Work out the finished part from the listing and answer in its coordinate system (mm). A direction names the side the tool comes from. Round coordinates to 2 decimals unless told otherwise and drop trailing zeros. Write each loop counter-clockwise with the first axis right and the second up, starting at its lowest first coordinate (ties: lowest second). Pieces come first, ordered by that corner, then holes. Notation, with made-up numbers: (-37.5, 13) -> (10.5, 13) arc R19 ccw to (10.5, 36) -> close; hole circle Ø6 at (54, -39.75). An arc over 180 degrees is marked (long way). One line per question, with ' | ' between items. Start each with the question number.
```python
from build123d import *

# Parameters (mm, degrees)
ESQUISSE1_W             = 41.6
ESQUISSE1_H             = 40
BOSS_EXTRU_1_DEPTH      = 4
BOSS_EXTRU_2_DEPTH      = 20
ESQUISSE3_R             = 19
ENL_V_MAT_EXTRU_1_DEPTH = 15
ENL_V_MAT_EXTRU_2_REACH = 62.626
ESQUISSE5_R             = 7
BOSS_EXTRU_3_DEPTH      = 6
D_GAGEMENT_M31_D        = 3.6
CONG_1_R                = 10
D_GAGEMENT_M32_D        = 3.6
ENL_V_MAT_EXTRU_3_DEPTH = 2.4
CONG_2_R                = 2


with BuildPart() as part:
    # Esquisse1 → Boss.-Extru.1 (new body)
    with BuildSketch(Plane(origin=(0, 0, 0), x_dir=(1, 0, 0), z_dir=(0, 1, 0))):
        with Locations((20.8, 0)):
            Rectangle(ESQUISSE1_W, ESQUISSE1_H)
    extrude(amount=BOSS_EXTRU_1_DEPTH)

    # Esquisse2 → Boss.-Extru.2 (add)
    with BuildSketch(Plane.ZY):
        with BuildLine():
            Line((-20, 4), (20, 4))
            Line((20, 4), (20, 24))
            ThreePointArc((20, 24), (0, 44), (-20, 24))
            Line((-20, 24), (-20, 4))
        make_face()
    extrude(amount=-BOSS_EXTRU_2_DEPTH)

    # Esquisse3 → Enlèv. mat.-Extru.1 (cut)
    with BuildSketch(Plane(origin=(20, 0, 0), x_dir=(0, 0, -1), z_dir=(1, 0, 0))):
        with Locations((0, 24)):
            Circle(ESQUISSE3_R)
    extrude(amount=-ENL_V_MAT_EXTRU_1_DEPTH, mode=Mode.SUBTRACT)

    # Esquisse5 → Enlèv. mat.-Extru.2 (cut, up to next)
    with BuildSketch(Plane(origin=(5, 0, 0), x_dir=(0, 0, -1), z_dir=(1, 0, 0)), mode=Mode.PRIVATE) as enl_v_mat_extru_2_sk1:
        with Locations((0, 17)):
            Circle(ESQUISSE5_R)
    enl_v_mat_extru_2_tool1 = extrude(enl_v_mat_extru_2_sk1.sketch, amount=-ENL_V_MAT_EXTRU_2_REACH, mode=Mode.PRIVATE) & part.part
    add(enl_v_mat_extru_2_tool1.solids().sort_by_distance((5, 17, 0))[0], mode=Mode.SUBTRACT)

    # Esquisse6 → Boss.-Extru.3 (add)
    with BuildSketch(Plane.XZ):
        with BuildLine():
            Line((3.5, 10), (3.5, -10))
            ThreePointArc((3.5, -10), (1.75, -11.75), (0, -10))
            Line((0, -10), (0, 10))
            ThreePointArc((0, 10), (1.75, 11.75), (3.5, 10))
        make_face()
        with BuildLine():
            Line((41.6, 10), (41.6, -10))
            ThreePointArc((41.6, -10), (39.85, -11.75), (38.1, -10))
            Line((38.1, -10), (38.1, 10))
            ThreePointArc((38.1, 10), (39.85, 11.75), (41.6, 10))
        make_face()
    extrude(amount=BOSS_EXTRU_3_DEPTH)

    # Dégagement M31 (through all)
    with Locations(Plane(origin=(5, 0, 0), x_dir=(0, 0, -1), z_dir=(1, 0, 0))):
        with Locations((-15.5, 24), (-7.75, 37.423393759), (7.75, 37.423393759), (15.5, 24), (7.75, 10.576606241), (-7.75, 10.576606241)):
            Hole(D_GAGEMENT_M31_D / 2)

    # Congé1
    cong_1_edges = [part.edges().sort_by_distance(p)[0] for p in [
        (41.6, 2, -20),
        (41.6, 2, 20),
    ]]
    fillet(cong_1_edges, radius=CONG_1_R)

    # Dégagement M32 (through all)
    with Locations(Plane(origin=(0, 4, 0), x_dir=(1, 0, 0), z_dir=(0, 1, 0))):
        with Locations((27.15, -15), (27.15, 15)):
            Hole(D_GAGEMENT_M32_D / 2)

    # Esquisse12 → Enlèv. mat.-Extru.3 (cut)
    with BuildSketch(Plane(origin=(0, 4, 0), x_dir=(1, 0, 0), z_dir=(0, 1, 0))):
        Polygon((30.036751346, -15), (28.593375673, -12.5), (25.706624327, -12.5), (24.263248654, -15), (25.706624327, -17.5), (28.593375673, -17.5), align=None)
        Polygon((30.036751346, 15), (28.593375673, 17.5), (25.706624327, 17.5), (24.263248654, 15), (25.706624327, 12.5), (28.593375673, 12.5), align=None)
    extrude(amount=-ENL_V_MAT_EXTRU_3_DEPTH, mode=Mode.SUBTRACT)

    # Congé2
    cong_2_edges = [part.edges().sort_by_distance(p)[0] for p in [
        (20, 4, 0),
    ]]
    fillet(cong_2_edges, radius=CONG_2_R)


solid = part.part
```
(1) The mould has two halves that part along X. Classify faces 1 (the flat face through (0, 25, 0)), 2 (the flat face through (27, 3, 17.5)), 3 (the flat face through (12, 12, -20)): +X half, -X half, draft (parallel to the pull), parting line (faces both ways), or undercut.
(2) Consider L1, parallel to X at y = 34, z = -5; L2, parallel to Y at x = 25, z = -7; L3, parallel to Y at x = 15, z = 17.5. Determine where each line is inside the solid, lowest interval first.
(3) A cutting plane is placed at C-C, the plane z = -7.75. Determine the outline of the cut face in (x, y).
(4) Given pin 1 Ø6 at (y, z) = (35, 12.5) entering from +X; pin 2 Ø6 at (y, z) = (37.42, 7.75) entering from -X; pin 3 Ø2 at (x, z) = (6, -3.5) entering from -Y; pin 4 Ø3 at (x, z) = (14, 3.5) entering from +Y, each flat-ended and moving along its own axis, determine where each tip first touches the part or whether it passes through.
(5) A cutting plane is placed at D-D, the plane x = 39.85. Determine the outline of the cut face in (y, z).
(6) For faces 4 (the flat face through (3.5, -3, 0)), 5 (the cylindrical face through (1.79, -2.96, -11.75)), 6 (the flat face through (29.305, 2.817, 16.267)), determine the directions among +Z, -Z, +X, -X, +Y, -Y from which every point of the face is accessible in a straight line to the end or side of a thin tool.
(7) A cutting plane is placed at A-A, the plane x = 8.5. Determine the outline of the cut face in (y, z), then the cut area to 3 significant figures.
(8) A cutting plane is placed at B-B, the plane y = 11.5. Determine the outline of the cut face in (x, z), then the cut area to 3 significant figures.
Returned:
1) face 1: -X half | face 2: undercut | face 3: draft
2) L1: 0 to 5 | L2: 0 to 4 | L3: 0 to 16.6, 31.4 to 33.68
3) outline: (0, -6) -> (3.5, -6) -> (3.5, 0) -> (38.1, 0) -> (38.1, -6) -> (41.6, -6) -> (41.6, 4) -> (22, 4) arc R2 cw to (20, 6) -> (20, 6.65) -> (5, 6.65) -> (5, 8.78) -> (0, 8.78) -> close; (0, 12.38) -> (5, 12.38) -> (5, 35.62) -> (0, 35.62) -> close; (0, 39.22) -> (5, 39.22) -> (5, 41.35) -> (20, 41.35) -> (20, 42.44) -> (0, 42.44) -> close
4) pin 1: x = 20 | pin 2: x = 0 | pin 3: y = 0 | pin 4: y = 43.9
5) outline: (-6, -11.75) -> (0, -11.75) -> (0, -15.65) -> (4, -15.65) -> (4, 15.65) -> (0, 15.65) -> (0, 11.75) -> (-6, 11.75) -> close
6) face 4: +Z, -Z, -Y | face 5: -Z, -Y | face 6: +Y
7) outline: (0, -20) -> (24, -20) arc R20 ccw to (24, 20) -> (0, 20) -> close; hole circle Ø38 at (24, 0) | area: 454 mm2
8) outline: (0, -20) -> (20, -20) -> (20, -14.31) -> (5, -14.31) -> (5, -9.3) -> (0, -9.3) -> close; (0, -6.2) -> (5, -6.2) -> (5, -4.33) -> (0, -4.33) -> close; (0, 4.33) -> (5, 4.33) -> (5, 6.2) -> (0, 6.2) -> close; (0, 9.3) -> (5, 9.3) -> (5, 14.31) -> (20, 14.31) -> (20, 20) -> (0, 20) -> close | area: 297 mm2
